Answer from the drawing. Dimensions are ordinates in mm from the lowest x, y and z of the part. Give positions to 0.01 mm unless a question says otherwise; leave off trailing zeros. Write each loop counter-clockwise with the first axis right and the second up, starting at its lowest first coordinate (ties: lowest second). Pieces come first, ordered by that corner, then holes. Notation, with made-up numbers: (-7, 35.5) -> (46, 35.5) arc R18 cw to (46, 61.5) -> close; hole circle Ø2 at (10.5, 32). An arc over 180 degrees is marked (long way). Put each result on its own line as item: value. Start each with the question number.
1) A cutting plane is placed at C-C (z = 0.7). Write down the section's boundary in (x, y).
2) Find the intervals of material crossed by line 1 along X through (y, z) = (10.75, 0.55); line 2 along X through (y, z) = (14.75, 0.2); line 3 along Y through (x, z) = (30.5, 0.8), in increasing order. Write a range as from..to.
3) A cutting plane is placed at B-B (x = 24). Write down the section's boundary in (y, z), then the cut area to 3 significant figures.
4) A cutting plane is placed at D-D (y = 14). Write down the section's boundary in (x, z), then the cut area to 3 significant figures.
5) A cutting plane is placed at A-A (y = 8). Write down the section's boundary in (x, z), then the cut area to 3 significant figures.
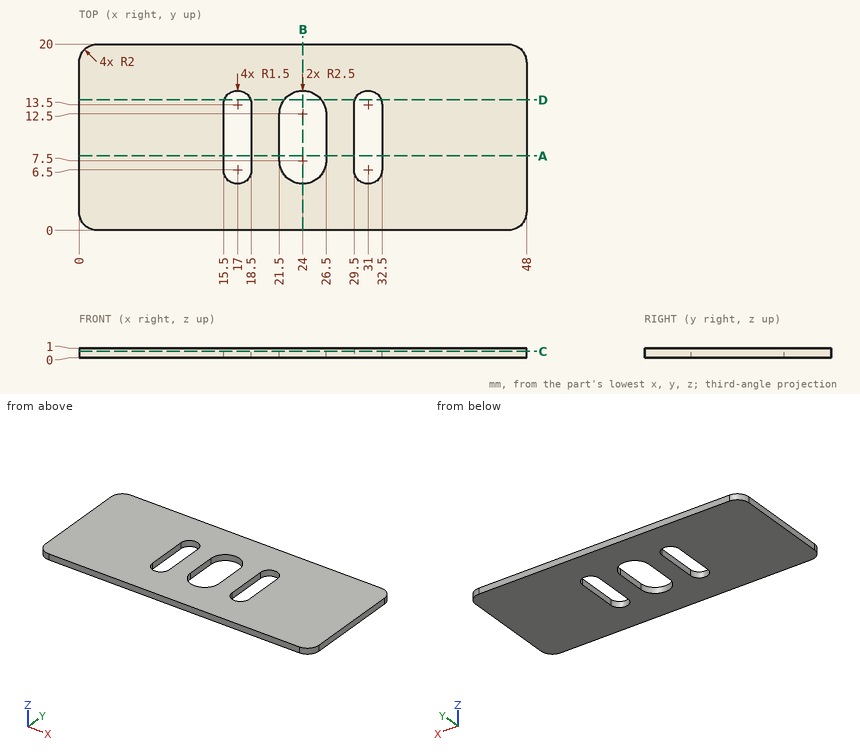
Reply:
1. outline: (0, 2) arc R2 ccw to (2, 0) -> (46, 0) arc R2 ccw to (48, 2) -> (48, 18) arc R2 ccw to (46, 20) -> (2, 20) arc R2 ccw to (0, 18) -> close; hole (15.5, 6.5) arc R1.5 ccw to (18.5, 6.5) -> (18.5, 13.5) arc R1.5 ccw to (15.5, 13.5) -> close; hole (21.5, 7.5) arc R2.5 ccw to (26.5, 7.5) -> (26.5, 12.5) arc R2.5 ccw to (21.5, 12.5) -> close; hole (29.5, 6.5) arc R1.5 ccw to (32.5, 6.5) -> (32.5, 13.5) arc R1.5 ccw to (29.5, 13.5) -> close
2. line 1: x = 0..15.5, 18.5..21.5, 26.5..29.5, 32.5..48
2. line 2: x = 0..16.17, 17.83..22.91, 25.09..30.17, 31.83..48
2. line 3: y = 0..5.09, 14.91..20
3. outline: (0, 0) -> (5, 0) -> (5, 1) -> (0, 1) -> close; (15, 0) -> (20, 0) -> (20, 1) -> (15, 1) -> close
3. area: 10.0 mm2
4. outline: (0, 0) -> (15.59, 0) -> (15.59, 1) -> (0, 1) -> close; (18.41, 0) -> (22, 0) -> (22, 1) -> (18.41, 1) -> close; (26, 0) -> (29.59, 0) -> (29.59, 1) -> (26, 1) -> close; (32.41, 0) -> (48, 0) -> (48, 1) -> (32.41, 1) -> close
4. area: 38.3 mm2
5. outline: (0, 0) -> (15.5, 0) -> (15.5, 1) -> (0, 1) -> close; (18.5, 0) -> (21.5, 0) -> (21.5, 1) -> (18.5, 1) -> close; (26.5, 0) -> (29.5, 0) -> (29.5, 1) -> (26.5, 1) -> close; (32.5, 0) -> (48, 0) -> (48, 1) -> (32.5, 1) -> close
5. area: 37.0 mm2
